```python
from build123d import *

# Parameters (mm, degrees)
F0_W     = 30
F0_H     = 30
F1_DEPTH = 2
F2_R     = 2
F3_DEPTH = 25
F2_W     = 30
F2_H     = 2
F4_DEPTH = 30
F5_R     = 2
F6_DEPTH = 25
F7_R     = 2.5


with BuildPart() as f1:
    # F0 (on Top) → F1 (new body)
    with BuildSketch(Plane.XY):
        Rectangle(F0_W, F0_H)
    extrude(amount=F1_DEPTH)

    # F2 (on face) → F3 (cut)
    with BuildSketch(Plane.XY.offset(2)):
        with Locations((0, 7)):
            Circle(F2_R)
        with Locations((0, -7)):
            Circle(F2_R)
    extrude(amount=-F3_DEPTH, mode=Mode.SUBTRACT)

    # F2 (on face) → F4 (join)
    with BuildSketch(Plane.XY.offset(2)):
        with Locations((0, 14)):
            Rectangle(F2_W, F2_H)
    extrude(amount=F4_DEPTH)

    # F5 (on face) → F6 (cut)
    with BuildSketch(Plane.XZ.offset(-13)):
        with Locations((0, 24)):
            Circle(F5_R)
        with Locations((0, 10)):
            Circle(F5_R)
    extrude(amount=-F6_DEPTH, mode=Mode.SUBTRACT)

    # F7
    f7_edges = [f1.edges().sort_by_distance(p)[0] for p in [
        (0, 15, 0),
    ]]
    fillet(f7_edges, radius=F7_R)


solid = f1.part
```
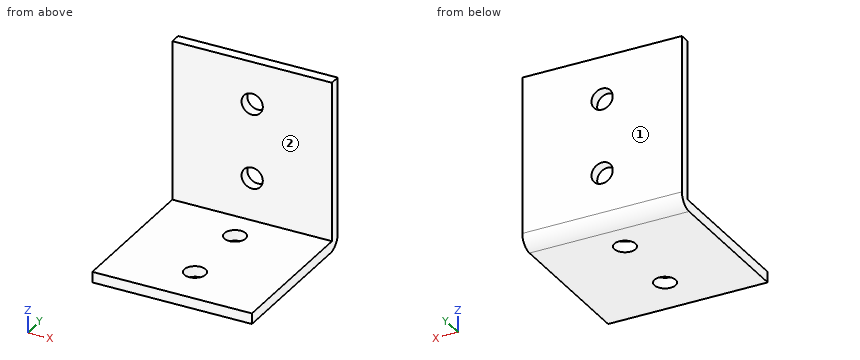
Can you work these out from the model? Positions are in its coordinate system, mm. Face numbers are marked on the shaded views. A direction names the side the tool comes from. Give positions to 0.01 mm unless a question says otherwise; leave off trailing zeros. Order: outer loops, then holes, each group sorted by start corner. A loop starts at its lowest first (then second) coordinate and runs counter-clockwise, first axis right, second up. Notation, with made-up numbers: (13.25, -7) - (46.25, -7) arc R34 cw to (46.25, 29) - close; hole circle Ø10 at (26, -32). An arc over 180 degrees is marked (long way). Use a Markdown table: item, result. Add a question column.
Q1. If we section it at C-C on x = 0: Write out the boundary of the cut face in (y, z), plus the area to 3 significant figures.
Q2. If we section it at D-D on x = 5.5: Write out the boundary of the cut face in (y, z), plus the area to 3 significant figures.
Q3. If we section it at A-A on z = 24: Write out the boundary of the cut face in (x, y), plus the area to 3 significant figures.
Q4. Please list where these lines run through material, in increasing order: line 1 along Y through (x, z) = (0, 1.5); line 2 along Z through (x, y) = (0, 14.2); line 3 along Y through (x, z) = (0, 1.1).
Q5. On a 3-axis mill with a long thin cutter (end or side, diameter ignored), from which of +Z, -Z, +X, -X, +Y, -Y can I reach the whole of each face in a straight line? I mean the marked faces 1 and 2. Say none if no direction works.
Q6. If we section it at B-B on y = 7: Write out the boundary of the cut face in (x, z), plus the area to 3 significant figures.
Q7. I'm going to push flat-ended pins straight in: pin 1 (3 mm diameter, centred on x = 4.5, y = 9.5, fed in from +Z); pin 2 (4.5 mm diameter, centred on x = 0, z = 10, fed in from -Y). Where does each tip first touch, or does it pass through?
Answers follow:
| question | item | result |
|---|---|---|
| 1 | outline | (-15, 0) - (-9, 0) - (-9, 2) - (-15, 2) - close; (-5, 0) - (5, 0) - (5, 2) - (-5, 2) - close; (9, 0) - (12.5, 0) arc R2.5 ccw to (15, 2.5) - (15, 8) - (13, 8) - (13, 2) - (9, 2) - close; (13, 12) - (15, 12) - (15, 22) - (13, 22) - close; (13, 26) - (15, 26) - (15, 32) - (13, 32) - close |
| 1 | area | 86.7 mm^2 |
| 2 | outline | (-15, 0) - (12.5, 0) arc R2.5 ccw to (15, 2.5) - (15, 32) - (13, 32) - (13, 2) - (-15, 2) - close |
| 2 | area | 119 mm^2 |
| 3 | outline | (-15, 13) - (-2, 13) - (-2, 15) - (-15, 15) - close; (2, 13) - (15, 13) - (15, 15) - (2, 15) - close |
| 3 | area | 52.0 mm^2 |
| 4 | line 1 | y = -15 to -9, -5 to 5, 9 to 14.79 |
| 4 | line 2 | z = 0.67 to 8, 12 to 22, 26 to 32 |
| 4 | line 3 | y = -15 to -9, -5 to 5, 9 to 14.57 |
| 5 | face 1 | +Z, -Z, +X, -X, +Y |
| 5 | face 2 | +Z, +X, -X, -Y |
| 6 | outline | (-15, 0) - (-2, 0) - (-2, 2) - (-15, 2) - close; (2, 0) - (15, 0) - (15, 2) - (2, 2) - close |
| 6 | area | 52.0 mm^2 |
| 7 | pin 1 | stops at z = 2 |
| 7 | pin 2 | stops at y = 13 |
